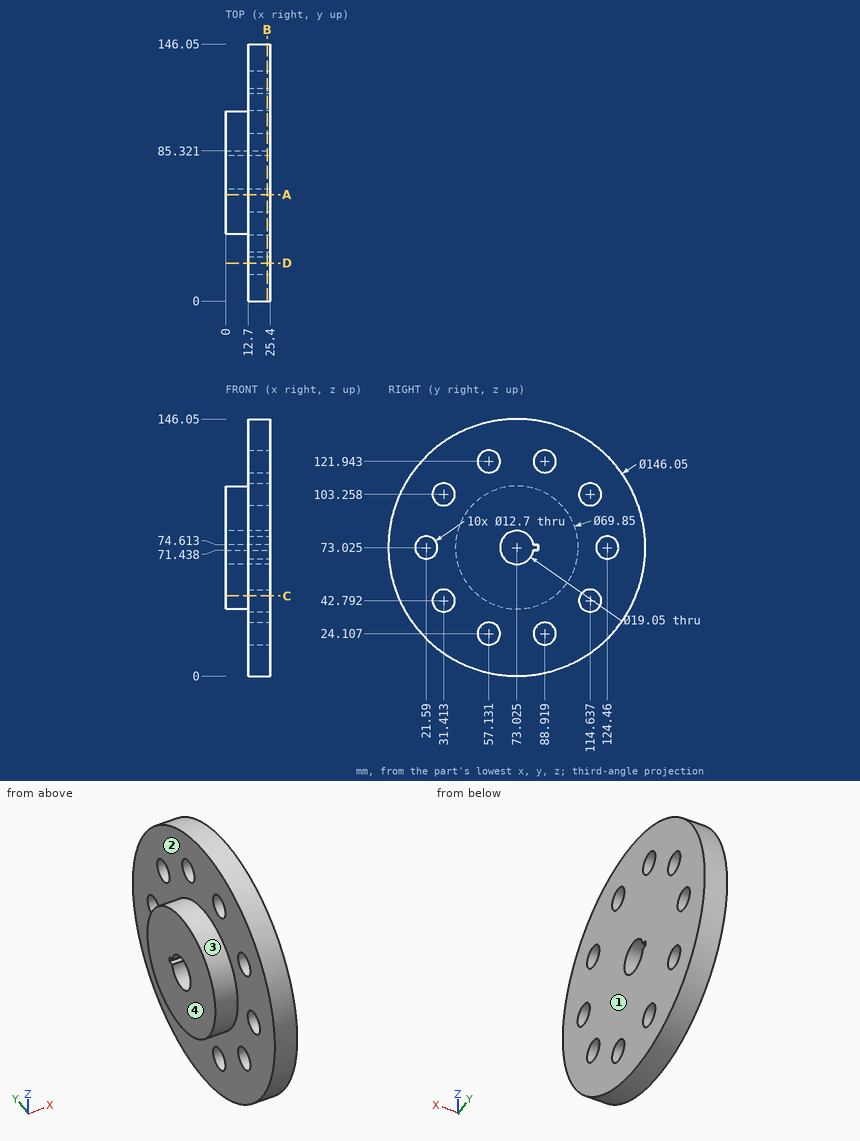
Verification items for this drawing (mm, ordinates from the low corner). A direction names the side the tool comes from. Coordinates: 2 decimals unless noted, no trailing zeros. Order: outer loops, then holes, each group sorted by start corner. A loop starts at its lowest first (then second) coordinate and runs counter-clockwise, first axis right, second up.
Q1. Sectioned sample at A-A on y = 60.5. Record the cut outline in (x, z) (1 decimal).
Reply:
outline: (0, 40.4) - (12.7, 40.4) - (12.7, 29.5) - (25.4, 29.5) - (25.4, 116.6) - (12.7, 116.6) - (12.7, 105.6) - (0, 105.6) - close; (12.7, 1.1) - (25.4, 1.1) - (25.4, 18.7) - (12.7, 18.7) - close; (12.7, 127.3) - (25.4, 127.3) - (25.4, 145) - (12.7, 145) - close
Q2. Sectioned sample at D-D on y = 21.59. Record the cut outline in (x, z) (1 decimal), and give its area (3 significant figures).
Reply:
outline: (12.7, 21.2) - (25.4, 21.2) - (25.4, 66.7) - (12.7, 66.7) - close; (12.7, 79.4) - (25.4, 79.4) - (25.4, 124.9) - (12.7, 124.9) - close
area: 1,160 mm2
Q3. Sectioned sample at B-B on x = 23.5. Give the number of separate pieces and of enclosed holes in the cut face, and give its area (3 significant figures).
Reply:
separate pieces: 1
enclosed holes: 11
area: 15,200 mm2
Q4. Depth check by flat-ended pin: pin 1 Ø20.5 at (y, z) = (31.41, 42.79) entering from -X; pin 2 Ø1.5 at (y, z) = (118.5, 38.5) entering from +X; pin 3 Ø11.5 at (y, z) = (114.64, 103.26) entering from +X; pin 4 Ø1.5 at (x, y) = (13, 96.5) entering from -Z (1 decimal). Enter the tip coordinate at first touch or a pass-through.
Reply:
pin 1: stops at x = 12.7
pin 2: stops at x = 25.4
pin 3: passes through
pin 4: stops at z = 3.6
Q5. Tool access check on the marked faces 1 and 2. Record the directions out of +Z, -Z, +X, -X, +Y, -Y that give a thin tool (end or side, any length) a straight path to the whole face; none if there is none.
Reply:
face 1: +Z, -Z, +X, +Y, -Y
face 2: -X
Q6. Draft check along Y on the marked faces 3 and 4. Enter one of: released by +Y, released by -Y, zero draft, split by the parting line, or undercut.
Reply:
face 3: split by the parting line
face 4: zero draft
Q7. Thickness scan on probe 1 along Y at (x, z) = (18.25, 77); probe 2 along X at (y, z) = (81.5, 128.5); probe 3 along Y at (x, z) = (15.5, 46) (1 decimal). Record the ranges inside material, lowest first.
Reply:
probe 1: y = 0.11 to 16.64, 26.54 to 64.37, 81.68 to 119.51, 129.41 to 145.94
probe 2: x = 12.7 to 25.4
probe 3: y = 5.2 to 25.9, 36.9 to 109.2, 120.1 to 140.9
Q8. Sectioned sample at C-C on z = 45.5. Record the cut outline in (x, y).
Reply:
outline: (0, 51.53) - (12.7, 51.53) - (12.7, 37.16) - (25.4, 37.16) - (25.4, 108.89) - (12.7, 108.89) - (12.7, 94.52) - (0, 94.52) - close; (12.7, 5.39) - (25.4, 5.39) - (25.4, 25.67) - (12.7, 25.67) - close; (12.7, 120.38) - (25.4, 120.38) - (25.4, 140.66) - (12.7, 140.66) - close
